Verification items for this drawing (mm, ordinates from the low corner). A direction names the side the tool comes from. Coordinates: 2 decimals unless noted, no trailing zeros. Loops run counter-clockwise (first coordinate to the right, second up) from the corner with the lowest first, then second, coordinate; pieces in that order, holes last. Notation, with made-up numbers: M -1.75,74.25 L 23.25,74.25 A22 cw 23.25,86.25 Z; hole C 47.25,32 d5. An arc over 180 degrees is marked long. Use CSV: the item, a comma, the result in double quotes.
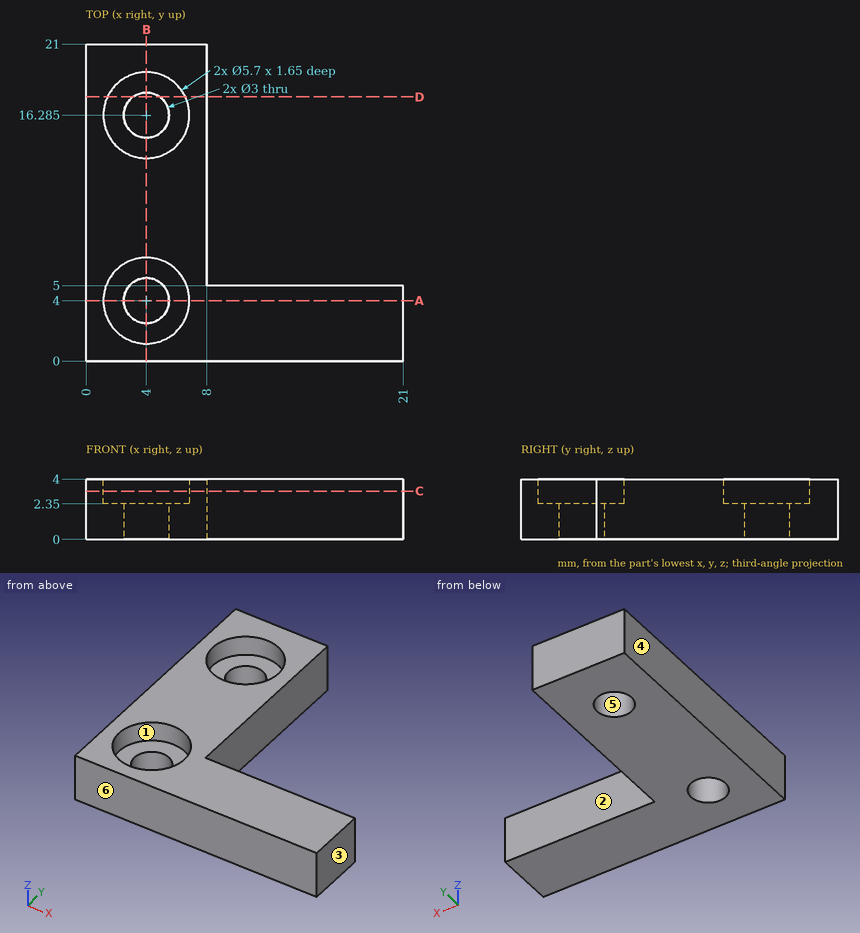
1. Section check D-D, the plane y = 17.5. Record the cut outline in (x, z).
The answers:
outline,"M 0,0 L 3.12,0 L 3.12,2.35 L 1.42,2.35 L 1.42,4 L 0,4 Z; M 4.88,0 L 8,0 L 8,4 L 6.58,4 L 6.58,2.35 L 4.88,2.35 Z"
2. Set-up check for the marked faces 1, 2 and 3: record each of +Z, -Z, +X, -X, +Y, -Y from which the full face is reachable in a straight line by a thin tool's end or side.
The answers:
face 1,"+Z"
face 2,"+Z, -Z, +X, +Y"
face 3,"+Z, -Z, +X, +Y, -Y"
3. Thickness scan on line 1 (Y direction, x = 4, z = 3.25) (3 decimals); line 2 (Y direction, x = 4, z = 1.8) (3 decimals); line 3 (X direction, y = 4, z = 1.55). Record the ranges inside material, lowest first. Write a range as [from, to].
The answers:
line 1,"[0, 1.15], [6.85, 13.435], [19.135, 21]"
line 2,"[0, 2.5], [5.5, 14.785], [17.785, 21]"
line 3,"[0, 2.5], [5.5, 21]"
4. Release check for a two-part mould opening along Y. For the marked faces 4, 5 and 6 record: +Y half, -Y half, draft (parallel to the pull), parting line (faces both ways), or undercut.
The answers:
face 4,"draft"
face 5,"undercut"
face 6,"-Y half"
5. Gauge pin test, flat ends, axial feed: P1, Ø1.2, axis at x = 12, z = 2, coming from the +Y side; P2, Ø4, axis at x = 11, y = 8, coming from the +Z side; P3, Ø1.7, axis at x = 3.5, y = 3.5, coming from the +Z side; P4, Ø2, axis at y = 11.5, z = 3, coming from the +X side. Record the tip position at first contact, or that the pin passes through.
The answers:
P1,"y = 5"
P2,"through"
P3,"z = 2.35"
P4,"x = 8"
6. Section check A-A, the plane y = 4. Record the cut outline in (x, z).
The answers:
outline,"M 0,0 L 2.5,0 L 2.5,2.35 L 1.15,2.35 L 1.15,4 L 0,4 Z; M 5.5,0 L 21,0 L 21,4 L 6.85,4 L 6.85,2.35 L 5.5,2.35 Z"
7. Section check B-B, the plane x = 4. Record the cut outline in (y, z) (3 decimals), plus the area to 3 significant figures.
The answers:
outline,"M 0,0 L 2.5,0 L 2.5,2.35 L 1.15,2.35 L 1.15,4 L 0,4 Z; M 5.5,0 L 14.785,0 L 14.785,2.35 L 13.435,2.35 L 13.435,4 L 6.85,4 L 6.85,2.35 L 5.5,2.35 Z; M 17.785,0 L 21,0 L 21,4 L 19.135,4 L 19.135,2.35 L 17.785,2.35 Z"
area,"51.1 mm^2"
8. Section check C-C, the plane z = 3.2. Record the cut outline in (x, y) (3 decimals).
The answers:
outline,"M 0,0 L 21,0 L 21,5 L 8,5 L 8,21 L 0,21 Z; hole C 4,4 d5.7; hole C 4,16.285 d5.7"
